Here's how the part is built. I have some questions about the finished solid (model axes, mm). Give positions to 0.01 mm unless a question says otherwise; leave off trailing zeros. Write each loop counter-clockwise with the first axis right and the second up, starting at its lowest first coordinate (ties: lowest second). Pieces come first, ordered by that corner, then holes. Notation, with made-up numbers: M -0.5,80.5 L 51.5,80.5 A13 cw 51.5,91.5 Z; hole C -28,79.5 d9. An arc over 180 degrees is marked long. Use one line per item in the form item = value. Start each with the question number.
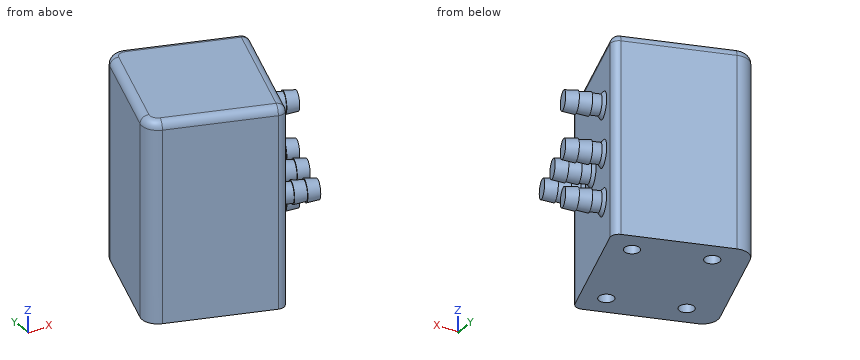
from build123d import *

# Parameters (mm, degrees)
BOSS_EXTRUDE1_DEPTH              = 79.642695409
FILLET1_R                        = 6.35
FILLET2_R                        = 3.175
SKETCH7_R                        = 4.261789822
CUT_EXTRUDE1_DEPTH               = 9.453613484
CHAMFER1_SIZE                    = 1.27
CHAMFER1_OF_SKETCH_PATTERN2_SIZE = 1.27
HOLE1_AT_2_COUNT                 = 2
HOLE1_AT_2_PITCH                 = 35.575698059
HOLE1_AT_3_COUNT                 = 2
HOLE1_AT_3_PITCH                 = 28.575
HOLE1_AT_4_COUNT                 = 2
HOLE1_AT_4_PITCH                 = 45.630701478
F_8_CLEARANCE_HOLE1_D            = 4.9149
F_8_CLEARANCE_HOLE1_DEPTH        = 12.7
F_8_CLEARANCE_HOLE1_TIP          = 1.476584928


with BuildPart() as part:
    # Sketch1 → Boss-Extrude1 (new body)
    with BuildSketch(Plane.XY):
        Polygon((290.280862854, 502.979981998), (307.307307279, 554.884385267), (355.576597736, 539.050383917), (338.550153311, 487.145980648), align=None)
    extrude(amount=BOSS_EXTRUDE1_DEPTH)

    # Fillet1
    fillet1_edges = [part.edges().sort_by_distance(p)[0] for p in [
        (307.307307279, 554.884385267, 39.821347704),
        (290.280862854, 502.979981998, 39.821347704),
    ]]
    fillet(fillet1_edges, radius=FILLET1_R)

    # Fillet2
    fillet2_edges = [part.edges().sort_by_distance(p)[0] for p in [
        (338.550153311, 487.145980648, 39.821347704),
        (298.794085066, 528.932183632, 79.642695409),
        (355.576597736, 539.050383917, 39.821347704),
        (317.432338736, 494.073356239, 79.642695409),
        (292.627790288, 504.167491527, 79.642695409),
        (308.494816808, 552.537457832, 79.642695409),
        (347.063375524, 513.098182283, 79.642695409),
        (334.458783161, 545.977759508, 79.642695409),
    ]]
    fillet(fillet2_edges, radius=FILLET2_R)

    # Sketch6 → Revolve1 (revolve)
    with BuildSketch(Plane.XY.offset(38.233847704), mode=Mode.PRIVATE) as revolve1_sk:
        Polygon((342.508653649, 499.213303263), (365.002143002, 491.834658634), (366.142191099, 495.310047547), (361.824191099, 497.311751702), (361.665851086, 496.829058798), (357.347851086, 498.830762953), (357.189511072, 498.348070049), (352.871511072, 500.349774204), (352.713171059, 499.8670813), (348.395171059, 501.868785456), (348.236831045, 501.386092551), (343.708665123, 502.87148802), align=None)
    revolve1 = revolve(revolve1_sk.sketch.rotate(Axis((342.508653649, 499.213303263, 38.233847704), (0.950182883020466, -0.31169293995038694, 0)), 180), axis=Axis((342.508653649, 499.213303263, 38.233847704), (0.950182883020466, -0.31169293995038694, 0)))

    # Sketch7 → Cut-Extrude1 (cut)
    with BuildSketch(Plane(origin=(183.876918982, -60.31800666, 0), x_dir=(0, 0, -1), z_dir=(0.9501828830204668, -0.31169293995038483, 0))):
        with Locations((-38.233847704, 581.101464951)):
            Circle(SKETCH7_R)
    cut_extrude1 = extrude(amount=-CUT_EXTRUDE1_DEPTH, mode=Mode.SUBTRACT)

    # Chamfer1
    chamfer1_edges = [part.edges().sort_by_distance(p)[0] for p in [
        (343.708665123, 502.87148802, 38.233847704),
    ]]
    chamfer(chamfer1_edges, length=CHAMFER1_SIZE)

    # Sketch-Pattern2: Revolve1, Cut-Extrude1 at 4 more places
    with Locations((9.109444, 27.769758, 0), (4.554722, 13.884879, 0), (9.109444, 27.769758, 19.116924), (9.109444, 27.769758, -19.116924)):
        add(revolve1)
        add(cut_extrude1, mode=Mode.SUBTRACT)

    # Chamfer1 of Sketch-Pattern2
    chamfer1_of_sketch_pattern2_edges = [part.edges().sort_by_distance(p)[0] for p in [
        (352.818109123, 530.64124602, 38.233847704),
        (348.263387123, 516.75636702, 38.233847704),
        (352.818109123, 530.64124602, 57.350771704),
        (352.818109123, 530.64124602, 19.116923704),
    ]]
    chamfer(chamfer1_of_sketch_pattern2_edges, length=CHAMFER1_OF_SKETCH_PATTERN2_SIZE)

    # Sketch9 → Hole1 (revolve, cut)
    with BuildSketch(Plane(origin=(332.468536604, 499.165347862, 0), x_dir=(0, 1, 0), z_dir=(1, 0, 0))):
        Polygon((0, 0), (0, 4.699), (2.8702, 4.699), (2.9972, 0), align=None)
    hole1 = revolve(axis=Axis((332.468536604, 499.165347862, 110), (0, 0, -1)), mode=Mode.SUBTRACT)

    # Hole1 at 2: Hole1 ×2
    with Locations(*[Vector(0.3116929399504022, 0.950182883020461, 0) * (i * HOLE1_AT_2_PITCH) for i in range(1, HOLE1_AT_2_COUNT)]):
        add(hole1, mode=Mode.SUBTRACT)

    # Hole1 at 3: Hole1 ×2
    with Locations(*[Vector(-0.9501828830204608, 0.3116929399504024, 0) * (i * HOLE1_AT_3_PITCH) for i in range(1, HOLE1_AT_3_COUNT)]):
        add(hole1, mode=Mode.SUBTRACT)

    # Hole1 at 4: Hole1 ×2
    with Locations(*[Vector(-0.3520169851244571, 0.9359936122559213, 0) * (i * HOLE1_AT_4_PITCH) for i in range(1, HOLE1_AT_4_COUNT)]):
        add(hole1, mode=Mode.SUBTRACT)

    # #8 Clearance Hole1
    with Locations(Plane(origin=(0, 0, 0), x_dir=(-1, 0, 0), z_dir=(0, 0, -1))):
        with Locations((-332.468536604, 499.165347862), (-343.557230523, 532.968767209), (-316.40575464, 541.875392969), (-305.317060721, 508.071973621)):
            Hole(F_8_CLEARANCE_HOLE1_D / 2, depth=F_8_CLEARANCE_HOLE1_DEPTH)
            with Locations((0, 0, -(F_8_CLEARANCE_HOLE1_DEPTH + F_8_CLEARANCE_HOLE1_TIP / 2))):  # 118° drill point
                Cone(0, F_8_CLEARANCE_HOLE1_D / 2, F_8_CLEARANCE_HOLE1_TIP, mode=Mode.SUBTRACT)


solid = part.part
1) Suppose I cut it at A-A, the plane z = 67. List the corners of the cut face in (x, y) for me (3 decimals), and give its area (3 significant figures).
2) Please list where these lines run through material, in increasing order: line 1 (Z direction, x = 295, y = 507); line 2 (X direction, y = 504, z = 18); line 3 (Y direction, x = 314, z = 30).
3) Will these pins go through, and if not, where does the flat tip stop? P1, Ø3, axis at x = 343.56, y = 532.97, coming from the -Z side; P2, Ø10, axis at y = 507, z = 47.5, coming from the +X side; P3, Ø8, axis at x = 354.5, z = 49.5, coming from the +Y side; P4, Ø4.5, axis at x = 315.5, y = 542, coming from the -Z side.
Checks:
q1.outline = M 292.26,509.014 A6.35 ccw 296.315,501.001 L 335.533,488.136 A3.175 ccw 339.54,490.163 L 354.587,536.034 A3.175 ccw 352.56,540.04 L 313.341,552.905 A6.35 ccw 305.328,548.851 Z
q1.area = 2,750 mm^2
q2.line_1 = 0 to 79.64
q2.line_2 = 292.72 to 344.08
q2.line_3 = 495.2 to 552.69
q3.P1 = 13.27
q3.P2 = 346.7
q3.P3 = 540.72
q3.P4 = 0
